The figure shows three views and two pictorial views of one solid part (mm, origin at its lowest corner). Answer the questions. Round coordinates to 2 decimals unless told otherwise and drop trailing zeros. Answer as CSV lines item,"result". Start each with the question number.
Item 1: Straight lines are drawn through the part: line 1 along X through (y, z) = (1.5, 25.5); line 2 along Z through (x, y) = (139.5, 4). For each, find the intervals that lie inside material, in ascending order. Write a range as [from, to].
Item 2: A cutting plane is placed at B-B on z = 32. State how many separate pieces and enclosed holes the cut face has, and give its area (3 significant figures).
Item 3: A flat-ended cylindrical pin translates along its axis: pin 1 (1 mm diameter, centred on y = 3.5, z = 6.5, fed in from -X). Find the tip coordinate at first contact, or state that the pin passes through.
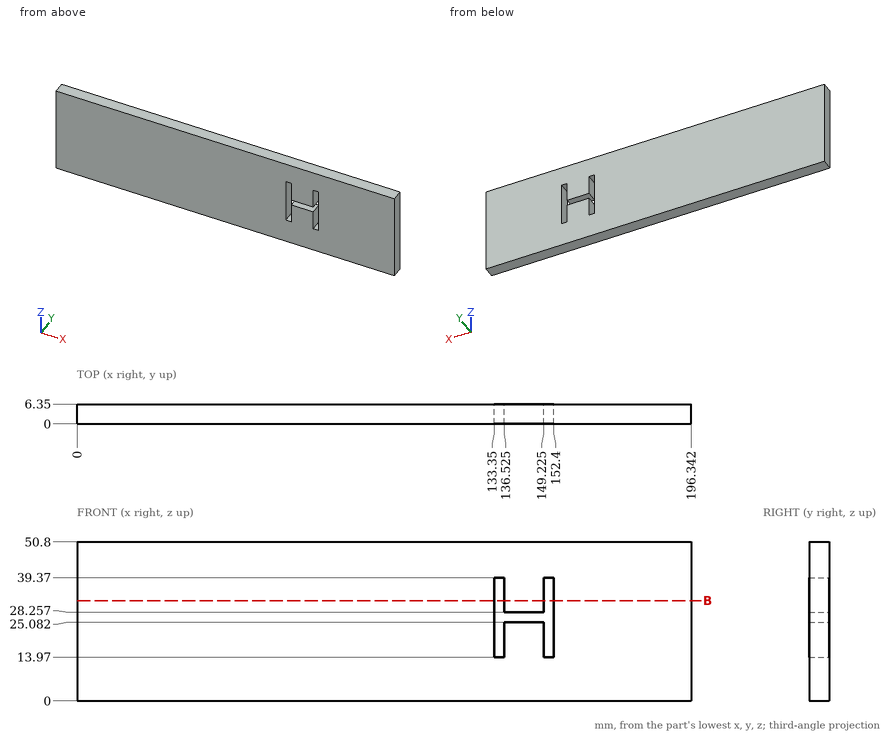
Geometry says:
1,line 1,"x = [0, 133.35], [152.4, 196.34]"
1,line 2,"z = [0, 25.08], [28.26, 50.8]"
2,separate pieces,"3"
2,enclosed holes,"0"
2,area,"1,210 mm^2"
3,pin 1,"stops at x = 0"
